```python
from build123d import *

# Parameters (mm, degrees)
BOSS_EXTRUDE1_DEPTH = 3
SKETCH2_W           = 120
SKETCH2_H           = 35
BOSS_EXTRUDE2_DEPTH = 12
CUT_EXTRUDE1_REACH  = 188.145
FILLET1_R           = 10
FILLET2_R           = 4
FILLET3_R           = 2


with BuildPart() as part:
    # Sketch1 → Boss-Extrude1 (new body)
    with BuildSketch(Plane.XY):
        with BuildLine():
            Line((180, 0), (180, -42))
            Line((180, -42), (0, -42))
            Line((0, -42), (0, 0))
            ThreePointArc((0, 0), (90, 22), (180, 0))
        make_face()
    extrude(amount=BOSS_EXTRUDE1_DEPTH)

    # Sketch2 → Boss-Extrude2 (add)
    with BuildSketch(Plane.XY.offset(3)):
        with Locations((90, -14.5)):
            Rectangle(SKETCH2_W, SKETCH2_H)
    extrude(amount=BOSS_EXTRUDE2_DEPTH)

    # Sketch3 → Cut-Extrude1 (cut, up to next)
    with BuildSketch(Plane(origin=(0, 3, 0), x_dir=(1, 0, 0), z_dir=(0, 1, 0)), mode=Mode.PRIVATE) as cut_extrude1_sk1:
        with BuildLine():
            Line((30, -15), (150, -15))
            ThreePointArc((150, -15), (90, -5.870751133), (30, -15))
        make_face()
    cut_extrude1_tool1 = extrude(cut_extrude1_sk1.sketch, amount=-CUT_EXTRUDE1_REACH, mode=Mode.PRIVATE) & part.part
    add(cut_extrude1_tool1.solids().sort_by_distance((90, 3, 11.341124))[0], mode=Mode.SUBTRACT)

    # Fillet1
    # the kernel refuses this fillet: 10 mm, written as the material it takes off along each edge
    with BuildSketch(Plane(origin=(150, 34.911423728, 15), x_dir=(0, 0, -1), z_dir=(0, -1, 0)), Plane(origin=(30, -63.911423728, 15), x_dir=(0, 0, -1), z_dir=(0, 1, 0))) as fillet1_piece_1:
        with BuildLine():
            CenterArc((13.125456564, -9.936465545), FILLET1_R, 96.462082414, 97.214818073)
            Line((3.409011311, -12.300929891), (3.214682406, -12.348219178))
            ThreePointArc((3.214682406, -12.348219178), (1.609086457, -6.176908891), (-0.190949181, -0.059484539))
            Line((-0.190949181, -0.059484539), (0, 0.2))
            ThreePointArc((0, 0.2), (6, 0.2), (11.977490869, 0.198729311))
            Line((11.977490869, 0.198729311), (12, 0))
        make_face()
    extrude(amount=98.822847456, mode=Mode.SUBTRACT)

    # Fillet2
    fillet2_edges = [part.edges().sort_by_distance(p)[0] for p in [
        (90, -32, 5.870751133),
        (90, 3, 5.870751133),
        (34.210640521, 3, 10.073014501),
        (145.789359479, 3, 10.073014501),
        (34.210640521, -32, 10.073014501),
        (145.789359479, -32, 10.073014501),
    ]]
    fillet(fillet2_edges, radius=FILLET2_R)

    # Fillet3
    # the kernel refuses this fillet: 2 mm, written as the material it takes off along each edge
    with BuildSketch(Plane(origin=(90, -173.090909091, 0), x_dir=(-0.4839116978541771, 0.8751168314458863, 0), z_dir=(-0.8751168314458863, -0.4839116978541771, 0))) as fillet3_piece_1:
        with BuildLine():
            CenterArc((195.090909091 - FILLET3_R, -FILLET3_R), FILLET3_R, 0, 90)
            Line((195.090909091 - FILLET3_R, 0), (195.090909091, 0))
            Line((195.090909091, 0), (195.090909091, -FILLET3_R))
        make_face()
    revolve(axis=Axis((90, -173.090909091, 0), (0, 0, -1)), revolution_arc=57.882388788, mode=Mode.SUBTRACT)
    with BuildSketch(Plane(origin=(90, -173.090909091, 3), x_dir=(-0.4839116978541771, 0.8751168314458863, 0), z_dir=(-0.8751168314458863, -0.4839116978541771, 0))) as fillet3_piece_2:
        with BuildLine():
            CenterArc((195.090909091 - FILLET3_R, FILLET3_R), FILLET3_R, 270, 90)
            Line((195.090909091, FILLET3_R), (195.090909091, 0))
            Line((195.090909091, 0), (195.090909091 - FILLET3_R, 0))
        make_face()
    revolve(axis=Axis((90, -173.090909091, 3), (0, 0, -1)), revolution_arc=57.882388788, mode=Mode.SUBTRACT)


solid = part.part
```
Here's how the part is built. I have some questions about the finished solid (model axes, mm). A direction names the side the tool comes from. Give positions to 0.01 mm unless a question says otherwise; leave off trailing zeros. Write each loop counter-clockwise with the first axis right and the second up, starting at its lowest first coordinate (ties: lowest second). Pieces come first, ordered by that corner, then holes. Notation, with made-up numbers: M 71,-17 L 103,-17 A13 ccw 103,-8 Z; hole C 37.5,30.25 d9. An arc over 180 degrees is marked long. Put each result on its own line as item: value. Start each with the question number.
Item 1: On a 3-axis mill with a long thin cutter (end or side, diameter ignored), from which of +Z, -Z, +X, -X, +Y, -Y can I reach the whole of each face in a straight line? I mean faces 1 (the flat face through (47, -32, 5)), 2 (the flat face through (91, -42, 1)), 3 (the flat face through (47, 3, 5)), 4 (the flat face through (91, -11, 0)), 5 (the flat face through (91.3, 3.2, 3)). Say none if no direction works.
Item 2: Thinking about a two-plate mould opening in X: for faces 6 (the cylindrical face through (90.67, -14.31, 5.87)), 7 (the flat face through (0, -21, 1)), 8 (the flat face through (180, -21, 1)), 9 (the flat face through (136, 3, 5)), which applies, +X half, -X half, draft (parallel to the pull), parting line (faces both ways), or undercut?
Item 3: I need wall thicknesses on L1, parallel to Z at x = 48, y = -36; L2, parallel to Z at x = 136, y = -9; L3, parallel to Y at x = 44.5, z = 8. Which ranges of each line are inside material? Lowest first, please. Write a range as from..to.
Item 4: Will these pins go through, and if not, where does the flat tip stop? pin 1 (3 mm diameter, centred on x = 115.5, y = -34, fed in from +Z); pin 2 (5.5 mm diameter, centred on x = 136, z = 5, fed in from +Y); pin 3 (2.5 mm diameter, centred on x = 58.5, z = 6, fed in from +Y).
Item 5: If we section it at A-A, the plane y = -13.5: Write out the boundary of the cut face in (x, z).
Values:
1. face 1: +Z, +X, -X, -Y
1. face 2: +Z, -Z, +X, -X, -Y
1. face 3: +Z, +X, -X, +Y
1. face 4: -Z, +X, -X, +Y, -Y
1. face 5: +Z
2. face 6: undercut
2. face 7: -X half
2. face 8: +X half
2. face 9: draft
3. L1: 0..3
3. L2: 0..11.19
3. L3: -31.87..2.87
4. pin 1: z = 3
4. pin 2: y = 16.14
4. pin 3: y = 2.98
5. outline: M 0,0 L 180,0 L 180,3 L 150,3 A10 ccw 137.7,11.59 A201.73 cw 42.3,11.59 A10 ccw 30,3 L 0,3 Z
